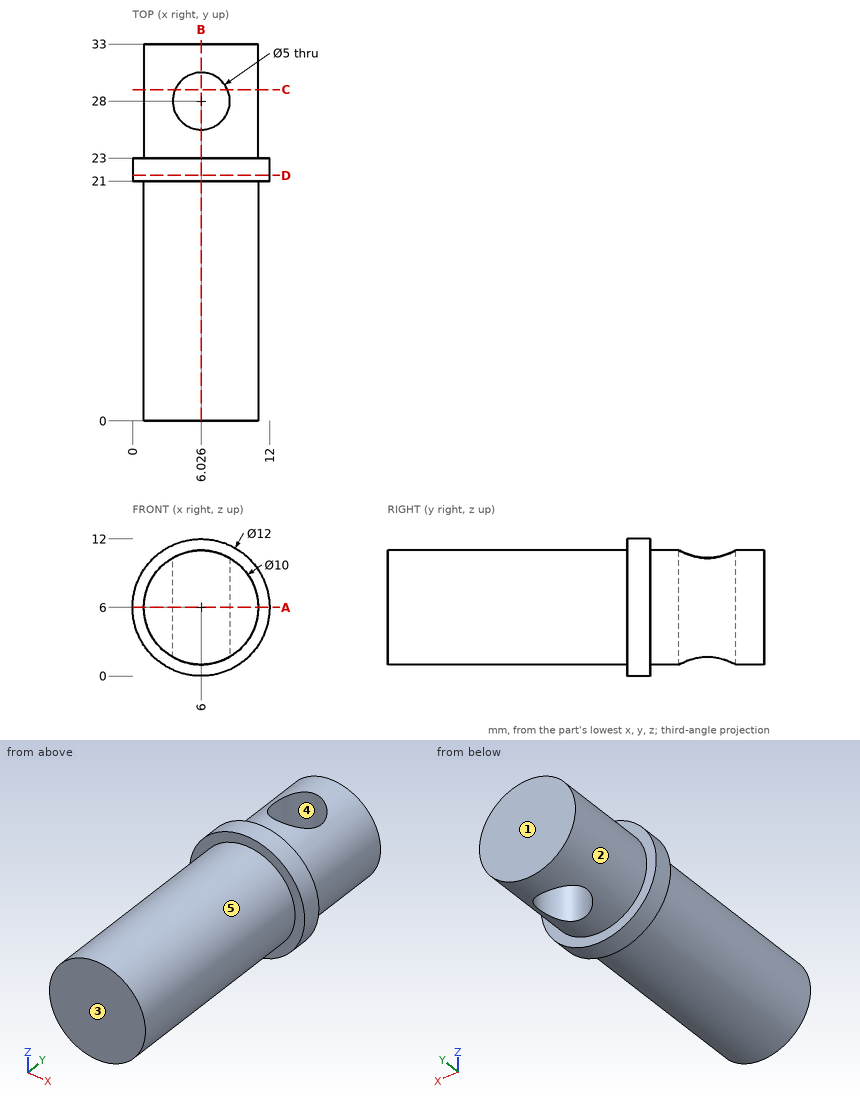
Check sheet for the drawn part. Datum: minimum x, y, z corner. Units: mm. A direction names the side the tool comes from. Coordinates: 2 decimals unless noted, no trailing zeros. Loops run counter-clockwise (first coordinate to the right, second up) from the corner with the lowest first, then second, coordinate; pieces in that order, holes last. Notation, with made-up numbers: M 51,52 L 91,52 A25 cw 91,81 Z; hole C 86.25,76 d4. An arc over 180 degrees is marked long. Answer as a JSON object with one key per item and string values.
1. Sectioned sample at B-B on x = 6. Record the cut outline in (y, z).
Outcome:
{"outline": "M 0,1 L 21,1 L 21,0 L 23,0 L 23,1 L 25.5,1 L 25.5,11 L 23,11 L 23,12 L 21,12 L 21,11 L 0,11 Z; M 30.5,1 L 33,1 L 33,11 L 30.5,11 Z"}
2. Sectioned sample at A-A on z = 6. Record the cut outline in (x, y) (1 decimal), and give its area (3 significant figures).
Outcome:
{"outline": "M 0,21 L 1,21 L 1,0 L 11,0 L 11,21 L 12,21 L 12,23 L 11,23 L 11,33 L 1,33 L 1,23 L 0,23 Z; hole C 6,28 d5", "area": "314 mm²"}
3. Release check for a two-part mould opening along Y. For the marked faces 3, 4 and 5 record: pulls with the +Y half, pulls with the -Y half, needs draft (parallel to the pull), parting line crosses it, or undercut.
Outcome:
{"face 3": "pulls with the -Y half", "face 4": "undercut", "face 5": "needs draft"}
4. Access from +Z, -Z, +X, -X, +Y, -Y to the whole of each face (thin tool, end or side, straight path). Record for the marked faces 1 and 2.
Outcome:
{"face 1": "+Z, -Z, +X, -X, +Y", "face 2": "+Y"}
5. Scan lines: L1, parallel to X at y = 28, z = 6 (1 decimal); L2, parallel to Y at x = 0.75, z = 8; L3, parallel to Z at x = 5.75, y = 23.5. Record each from-to range of solid material in increasing order. Write a range as from..to.
Outcome:
{"L1": "1..3.5, 8.5..11", "L2": "21..23", "L3": "1.01..10.99"}
6. Sectioned sample at D-D on y = 21.5. Record the cut outline in (x, z), and give its area (3 significant figures).
Outcome:
{"outline": "C 6,6 d12", "area": "113 mm²"}
7. Sectioned sample at C-C on y = 29. Record the cut outline in (x, z) (1 decimal).
Outcome:
{"outline": "M 3.7,1.5 L 3.7,10.5 A5 ccw Z; M 8.3,1.6 A5 ccw 8.3,10.4 Z"}
8. Depth check by flat-ended pin: P1, Ø3, axis at y = 14.5, z = 3, coming from the +X side; P2, Ø1, axis at x = 1, y = 3.5, coming from the +Z side; P3, Ø4, axis at x = 6.03, y = 28, coming from the +Z side; P4, Ø3, axis at y = 13, z = 4, coming from the -X side (1 decimal). Enter the tip coordinate at first touch or a pass-through.
Outcome:
{"P1": "x = 10.77", "P2": "z = 8.18", "P3": "through", "P4": "x = 1"}
